from build123d import *

# Parameters (mm, degrees)
F2_W      = 40
F2_H      = 60
F3_DEPTH  = 148.5
F4_T      = -2
F5_W      = 36
F5_H      = 31
F6_DEPTH  = 2
F7_R      = 4.5
F8_DEPTH  = 40.001
F9_R      = 4.5
F10_DEPTH = 60.001
F9_R_2    = 8
F11_DEPTH = 2


with BuildPart() as f3:
    # F2 (on Top) → F3 (new body)
    with BuildSketch(Plane.XY):
        with Locations((-20, -30)):
            Rectangle(F2_W, F2_H)
    extrude(amount=F3_DEPTH)

    # F4
    f4_openings = [f3.faces().sort_by_distance(p)[0] for p in [
        (-20, -30, 148.5),
        (-20, -30, 0),
    ]]
    offset(amount=F4_T, openings=f4_openings)

    # F5 (on face) → F6 (cut, through all)
    with BuildSketch(Plane(origin=(0, 0, 0), x_dir=(-1, 0, 0), z_dir=(0, 1, 0))):
        with Locations((20, 133)):
            Rectangle(F5_W, F5_H)
    extrude(amount=-F6_DEPTH, mode=Mode.SUBTRACT)

    # F7 (on Right) → F8 (cut, through all)
    with BuildSketch(Plane.YZ):
        with Locations((-30, 133)):
            Circle(F7_R)
    extrude(amount=-F8_DEPTH, mode=Mode.SUBTRACT)

    # F9 (on face) → F10 (cut, through all)
    with BuildSketch(Plane.XZ.offset(60)):
        with Locations((-20, 35)):
            Circle(F9_R)
        with Locations((-20, 15)):
            Circle(F9_R)
    extrude(amount=-F10_DEPTH, mode=Mode.SUBTRACT)

    # F9 (on face) → F11 (cut, through all)
    with BuildSketch(Plane.XZ.offset(60)):
        with Locations((-20, 35)):
            Circle(F9_R_2)
        with Locations((-20, 35)):
            Circle(F9_R, mode=Mode.SUBTRACT)
        with Locations((-20, 15)):
            Circle(F9_R_2)
        with Locations((-20, 15)):
            Circle(F9_R, mode=Mode.SUBTRACT)
    extrude(amount=-F11_DEPTH, mode=Mode.SUBTRACT)


solid = f3.part
Source: CAD feature listing. Evaluate the final solid. Frame: model axes, mm. A direction names the side the tool comes from. Round coordinates to 2 decimals unless told otherwise and drop trailing zeros. Write each loop counter-clockwise with the first axis right and the second up, starting at its lowest first coordinate (ties: lowest second). Pieces come first, ordered by that corner, then holes. Notation, with made-up numbers: M 26.5,67.5 L 42.5,67.5 A8 ccw 42.5,81.5 Z; hole C -15.75,36 d7. An arc over 180 degrees is marked long. One line per item, written item: value. Start each with the question number.
Item 1: Set-up query: faces 4 (the cylindrical face through (-23.32, -1.01, 18.04)), 5 (the cylindrical face through (-21.041, -59.014, 42.932)), 6 (the flat face through (-20, -2, 58)). Return all of +Z, -Z, +X, -X, +Y, -Y with unobstructed straight access to the full face (end or side cutting, diameter ignored); none if empty.
Item 2: Pin query (flat end, axial travel): pin 1 (1 mm diameter, centred on x = -16.5, y = -1, fed in from +Z); pin 2 (14.5 mm diameter, centred on x = -20, z = 35, fed in from -Y). Return the tip coordinate at first contact, or that it passes through.
Item 3: Section query D-D (y = -30). Return the cut outline in (x, z), plus the area to 3 significant figures.
Item 4: Ray query, L1, parallel to Z at x = -20, y = -0.65; L2, parallel to Z at x = -20, y = -58.55; L3, parallel to X at y = -31, z = 71.5. Return the intervals inside material, ascending. Write a range as from..to.
Item 5: Section query C-C (x = -20). Return the cut outline in (y, z).
Item 6: Mould query, pull axis X, two halves, no side actions, for faces 1 (the flat face through (-39, -30, 0)), 2 (the cylindrical face through (-21.73, -59.01, 7.19)), 3 (the flat face through (-40, -30, 73)). Classes: pulls with the +X half, pulls with the -X half, needs draft (parallel to the pull), parting line crosses it, or undercut.
Item 7: Section query B-B (z = 35). Return the cut outline in (x, y).
Item 8: Section query A-A (z = 133). Return the cut outline in (x, y).
Result set:
1. face 4: +Y, -Y
1. face 5: -Y
1. face 6: +Z, -Z
2. pin 1: stops at z = 117.5
2. pin 2: stops at y = -2
3. outline: M -40,0 L -38,0 L -38,128.5 L -40,128.5 Z; M -40,137.5 L -38,137.5 L -38,148.5 L -40,148.5 Z; M -2,0 L 0,0 L 0,128.5 L -2,128.5 Z; M -2,137.5 L 0,137.5 L 0,148.5 L -2,148.5 Z
3. area: 558 mm²
4. L1: z = 0..10.5, 19.5..30.5, 39.5..117.5
4. L2: z = 0..7, 23..27, 43..148.5
4. L3: x = -40..-38, -2..0
5. outline: M -60,0 L -58,0 L -58,7 L -60,7 Z; M -60,23 L -58,23 L -58,27 L -60,27 Z; M -60,43 L -58,43 L -58,148.5 L -60,148.5 Z; M -2,0 L 0,0 L 0,10.5 L -2,10.5 Z; M -2,19.5 L 0,19.5 L 0,30.5 L -2,30.5 Z; M -2,39.5 L 0,39.5 L 0,117.5 L -2,117.5 Z
6. face 1: needs draft
6. face 2: undercut
6. face 3: pulls with the -X half
7. outline: M -40,-60 L -28,-60 L -28,-58 L -38,-58 L -38,-2 L -24.5,-2 L -24.5,0 L -40,0 Z; M -15.5,-2 L -2,-2 L -2,-58 L -12,-58 L -12,-60 L 0,-60 L 0,0 L -15.5,0 Z
8. outline: M -40,-60 L 0,-60 L 0,-34.5 L -2,-34.5 L -2,-58 L -38,-58 L -38,-34.5 L -40,-34.5 Z; M -40,-25.5 L -38,-25.5 L -38,0 L -40,0 Z; M -2,-25.5 L 0,-25.5 L 0,0 L -2,0 Z
